from build123d import *

# Parameters (mm, degrees)
ESBO_O1_R                = 1.6
RESSALTO_EXTRUS_O1_DEPTH = 0.75
CORTE_EXTRUS_O1_REACH    = 123.445
ESBO_O2_R                = 4
ESBO_O2_R_2              = 1.1


with BuildPart() as part:
    # Esboço1 → Ressalto-extrusão1 (new, symmetric)
    with BuildSketch(Plane(origin=(0, 0, 0), x_dir=(1, 0, 0), z_dir=(0, 1, 0))):
        with BuildLine():
            ThreePointArc((-33.25966317, 13.776603565), (-36, 0), (-33.25966317, -13.776603565))
            ThreePointArc((-33.25966317, -13.776603565), (-33.583097891, -17.060491394), (-36.493241534, -18.615995578))
            ThreePointArc((-36.493241534, -18.615995578), (-72.090991916, -8.566197582), (-109, -11))
            ThreePointArc((-109, -11), (-120, 0), (-109, 11))
            ThreePointArc((-109, 11), (-72.090991916, 8.566197582), (-36.493241534, 18.615995578))
            ThreePointArc((-36.493241534, 18.615995578), (-33.583097891, 17.060491394), (-33.25966317, 13.776603565))
        make_face()
        with Locations(Location((-36.493241534, 15.115995578, 0), (0, 0, 270))):
            Circle(ESBO_O1_R, mode=Mode.SUBTRACT)
        with Locations(Location((-36.493241534, -15.115995578, 0), (0, 0, 270))):
            Circle(ESBO_O1_R, mode=Mode.SUBTRACT)
        with Locations(Location((-95.79, 6, 0), (0, 0, 270))):
            Circle(ESBO_O1_R, mode=Mode.SUBTRACT)
        with Locations(Location((-95.79, -5.96, 0), (0, 0, 270))):
            Circle(ESBO_O1_R, mode=Mode.SUBTRACT)
    extrude(amount=RESSALTO_EXTRUS_O1_DEPTH, both=True)

    # Esboço2 → Corte-extrusão1 (cut, up to next)
    with BuildSketch(Plane(origin=(0, 0.75, 0), x_dir=(1, 0, 0), z_dir=(0, 1, 0)), mode=Mode.PRIVATE) as corte_extrus_o1_sk1:
        with Locations(Location((-109, 0, 0), (0, 0, 270))):
            Circle(ESBO_O2_R)
    corte_extrus_o1_tool1 = extrude(corte_extrus_o1_sk1.sketch, amount=-CORTE_EXTRUS_O1_REACH, mode=Mode.PRIVATE) & part.part
    # Esboço2 → Corte-extrusão1 (cut, up to next)
    with BuildSketch(Plane(origin=(0, 0.75, 0), x_dir=(1, 0, 0), z_dir=(0, 1, 0)), mode=Mode.PRIVATE) as corte_extrus_o1_sk2:
        with Locations(Location((-103.586557067, 5.545911613, 0), (0, 0, 270))):
            Circle(ESBO_O2_R_2)
    corte_extrus_o1_tool2 = extrude(corte_extrus_o1_sk2.sketch, amount=-CORTE_EXTRUS_O1_REACH, mode=Mode.PRIVATE) & part.part
    # Esboço2 → Corte-extrusão1 (cut, up to next)
    with BuildSketch(Plane(origin=(0, 0.75, 0), x_dir=(1, 0, 0), z_dir=(0, 1, 0)), mode=Mode.PRIVATE) as corte_extrus_o1_sk3:
        with Locations(Location((-103.454088387, -5.413442933, 0), (0, 0, 270))):
            Circle(ESBO_O2_R_2)
    corte_extrus_o1_tool3 = extrude(corte_extrus_o1_sk3.sketch, amount=-CORTE_EXTRUS_O1_REACH, mode=Mode.PRIVATE) & part.part
    # Esboço2 → Corte-extrusão1 (cut, up to next)
    with BuildSketch(Plane(origin=(0, 0.75, 0), x_dir=(1, 0, 0), z_dir=(0, 1, 0)), mode=Mode.PRIVATE) as corte_extrus_o1_sk4:
        with Locations(Location((-114.413442933, -5.545911613, 0), (0, 0, 270))):
            Circle(ESBO_O2_R_2)
    corte_extrus_o1_tool4 = extrude(corte_extrus_o1_sk4.sketch, amount=-CORTE_EXTRUS_O1_REACH, mode=Mode.PRIVATE) & part.part
    # Esboço2 → Corte-extrusão1 (cut, up to next)
    with BuildSketch(Plane(origin=(0, 0.75, 0), x_dir=(1, 0, 0), z_dir=(0, 1, 0)), mode=Mode.PRIVATE) as corte_extrus_o1_sk5:
        with Locations(Location((-114.545911613, 5.413442933, 0), (0, 0, 270))):
            Circle(ESBO_O2_R_2)
    corte_extrus_o1_tool5 = extrude(corte_extrus_o1_sk5.sketch, amount=-CORTE_EXTRUS_O1_REACH, mode=Mode.PRIVATE) & part.part
    # Esboço2 → Corte-extrusão1 (cut, up to next)
    with BuildSketch(Plane(origin=(0, 0.75, 0), x_dir=(1, 0, 0), z_dir=(0, 1, 0)), mode=Mode.PRIVATE) as corte_extrus_o1_sk6:
        with BuildLine():
            Line((-88.078445949, 2.757577424), (-52.119636338, 7.831519885))
            ThreePointArc((-52.119636338, 7.831519885), (-44.288116453, 0), (-52.119636338, -7.831519885))
            Line((-52.119636338, -7.831519885), (-88.078445949, -2.757577424))
            ThreePointArc((-88.078445949, -2.757577424), (-90.836023373, 0), (-88.078445949, 2.757577424))
        make_face()
    corte_extrus_o1_tool6 = extrude(corte_extrus_o1_sk6.sketch, amount=-CORTE_EXTRUS_O1_REACH, mode=Mode.PRIVATE) & part.part
    add(corte_extrus_o1_tool1.solids().sort_by_distance((-109, 0.75, 0))[0], mode=Mode.SUBTRACT)
    add(corte_extrus_o1_tool2.solids().sort_by_distance((-103.586557, 0.75, -5.545912))[0], mode=Mode.SUBTRACT)
    add(corte_extrus_o1_tool3.solids().sort_by_distance((-103.454088, 0.75, 5.413443))[0], mode=Mode.SUBTRACT)
    add(corte_extrus_o1_tool4.solids().sort_by_distance((-114.413443, 0.75, 5.545912))[0], mode=Mode.SUBTRACT)
    add(corte_extrus_o1_tool5.solids().sort_by_distance((-114.545912, 0.75, -5.413443))[0], mode=Mode.SUBTRACT)
    add(corte_extrus_o1_tool6.solids().sort_by_distance((-64.134293, 0.75, 0))[0], mode=Mode.SUBTRACT)


solid = part.part
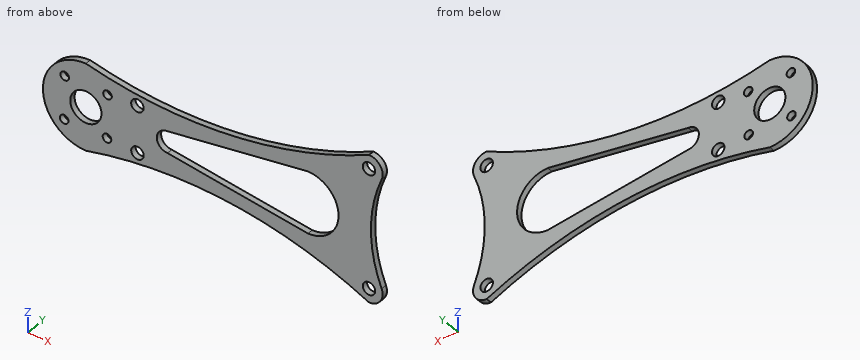
Here's how the part is built. I have some questions about the finished solid (model axes, mm). Coordinates: 2 decimals unless noted, no trailing zeros. Write each loop counter-clockwise with the first axis right and the second up, starting at its lowest first coordinate (ties: lowest second). Pieces come first, ordered by that corner, then holes.
Item 1: If I drill on line 1 (Z direction, x = -115, y = -0.35); line 2 (X direction, y = 0.05, z = 1); line 3 (Z direction, x = -97, y = -0.05), over which ranges is the centre line in solid material (lowest first)?
Item 2: I want a section at C-C on x = -95.79. Write out the boundary of the cut face in (y, z).
Item 3: Will this pin go through, and if not, where does the flat tip stop? pin 1 (3 mm diameter, centred on x = -114.55, z = -5.41, fed in from +Y).
Item 4: I want a section at D-D on y = -0.05. Count the separate pieces of the cut face and the enclosed holes in it, and give its area (3 significant figures).
Item 5: I want a section at A-A on x = -61.5. Write out the boundary of the cut face in (y, z), and give its area (3 significant figures).
Item 6: I want a section at B-B on z = -0.5. Write out the boundary of the cut face in (x, y), and give its area (3 significant figures).
Findings below:
1. line 1: z = -9.22 to -6.42, -4.41 to 4.62, 6.48 to 9.22
1. line 2: x = -119.95 to -112.87, -105.13 to -90.65, -44.35 to -35.99
1. line 3: z = -8.81 to -7.05, -4.95 to 4.91, 7.01 to 8.81
2. outline: (-0.75, -8.67) - (0.75, -8.67) - (0.75, -7.6) - (-0.75, -7.6) - close; (-0.75, -4.4) - (0.75, -4.4) - (0.75, 4.36) - (-0.75, 4.36) - close; (-0.75, 7.56) - (0.75, 7.56) - (0.75, 8.67) - (-0.75, 8.67) - close
3. pin 1: stops at y = 0.75
4. separate pieces: 1
4. enclosed holes: 10
4. area: 1,200 mm2
5. outline: (-0.75, -10.21) - (0.75, -10.21) - (0.75, -6.51) - (-0.75, -6.51) - close; (-0.75, 6.51) - (0.75, 6.51) - (0.75, 10.21) - (-0.75, 10.21) - close
5. area: 11.1 mm2
6. outline: (-119.99, -0.75) - (-112.97, -0.75) - (-112.97, 0.75) - (-119.99, 0.75) - close; (-105.03, -0.75) - (-90.79, -0.75) - (-90.79, 0.75) - (-105.03, 0.75) - close; (-44.3, -0.75) - (-36, -0.75) - (-36, 0.75) - (-44.3, 0.75) - close
6. area: 44.4 mm2
